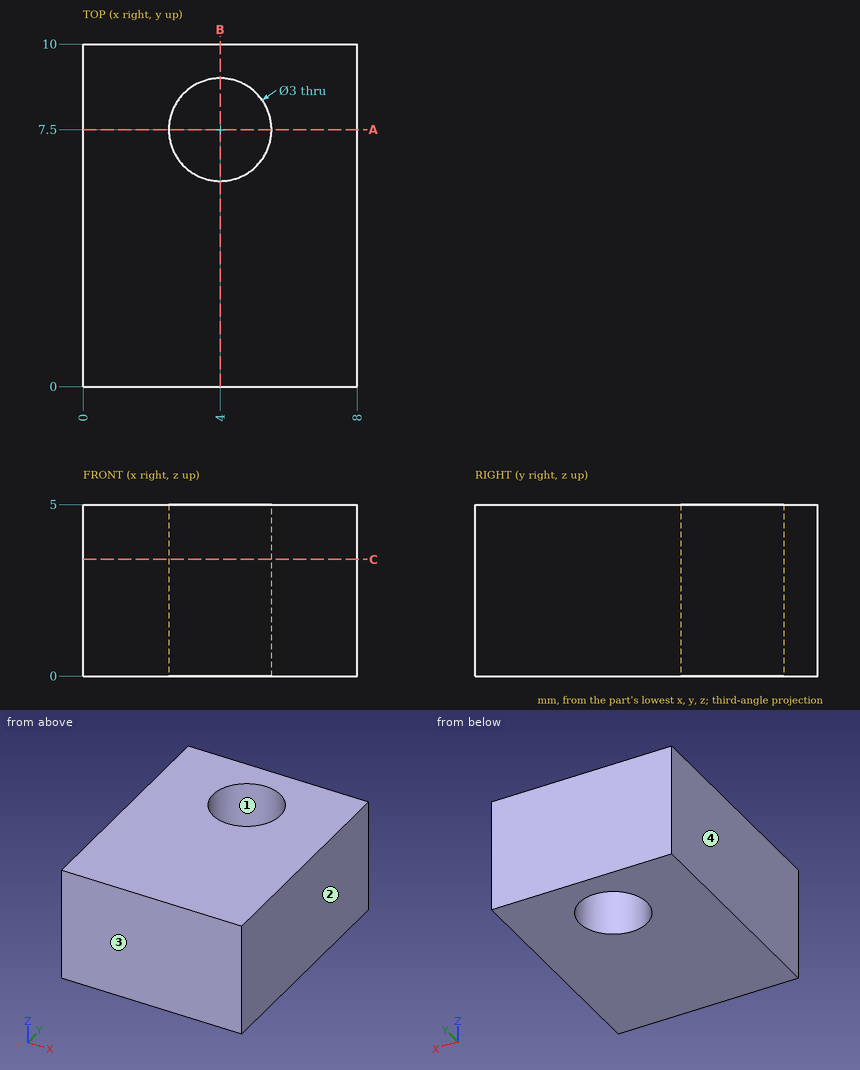
For this review, use the dimensioned drawing (mm, ordinates from the lowest corner) and the shaded views. Coordinates: 2 decimals unless noted, no trailing zeros. Order: outer loops, then holes, each group sorted by start corner. A loop starts at its lowest first (then second) coordinate and runs counter-clockwise, first axis right, second up. Notation, with made-up numbers: (48.5, 22.25) - (82.5, 22.25) arc R29 ccw to (82.5, 51.25) - close; hole circle Ø8 at (27, 30). An arc over 180 degrees is marked (long way). Answer as a JSON object with one key per item and string values. Group by question number.
1. For probe 1 along Y at (x, z) = (4, 1.2); probe 2 along Y at (x, z) = (3.5, 4.2); probe 3 along X at (y, z) = (8, 3.35), list the stretches that pass through material, from the lowest coordinate up.
2. We need section B-B on x = 4. State the section outline as (y, z) points.
3. We need section A-A on y = 7.5. State the section outline as (x, z) points.
4. We need section C-C on z = 3.4. State the section outline as (x, y) points.
5. The part is to be moulded in two halves that separate along X. For the marked faces 1, 2, 3 and 4, say which applies: pulls with the +X half, pulls with the -X half, needs draft (parallel to the pull), parting line crosses it, or undercut.
Final values:
{
 "1": {"probe 1": "0 to 6, 9 to 10", "probe 2": "0 to 6.09, 8.91 to 10", "probe 3": "0 to 2.59, 5.41 to 8"},
 "2": {"outline": "(0, 0) - (6, 0) - (6, 5) - (0, 5) - close; (9, 0) - (10, 0) - (10, 5) - (9, 5) - close"},
 "3": {"outline": "(0, 0) - (2.5, 0) - (2.5, 5) - (0, 5) - close; (5.5, 0) - (8, 0) - (8, 5) - (5.5, 5) - close"},
 "4": {"outline": "(0, 0) - (8, 0) - (8, 10) - (0, 10) - close; hole circle Ø3 at (4, 7.5)"},
 "5": {"face 1": "undercut", "face 2": "pulls with the +X half", "face 3": "needs draft", "face 4": "pulls with the -X half"}
}
